Build history of the part. All positions in model axes, mm. A direction names the side the tool comes from. Round coordinates to 2 decimals unless told otherwise and drop trailing zeros. Order: outer loops, then holes, each group sorted by start corner. A loop starts at its lowest first (then second) coordinate and runs counter-clockwise, first axis right, second up. Notation, with made-up numbers: (-21, 84.5) - (3, 84.5) arc R13 ccw to (3, 93.5) - close; hole circle Ø10 at (13, -11.75). An arc over 180 degrees is marked (long way). One line per question, with ' | ' between items. Start each with the question number.
Autodesk Inventor part; units mm, degrees
ref_plane "YZ Plane" through (0, 0, 0) normal (1, 0, 0) x (0, 1, 0)
ref_plane "XZ Plane" through (0, 0, 0) normal (0, 1, 0) x (-1, 0, 0)
ref_plane "XY Plane" through (0, 0, 0) normal (0, 0, 1) x (1, 0, 0)
sketch "Sketch1" plane through (0, 0, 0) normal (0, 1, 0) x (-1, 0, 0)
  circle A0 centre (7.3, 0) radius 1.55
  circle A1 centre (0, 0) radius 1.55
  line L0 (0, 10.8163) -> (0, -10.8163)
  line L1 (6.335, 0) -> (-6.335, 0)
  line L2 (-3.55, 12.16) -> (16.45, 12.16)
  line L3 (16.45, 12.16) -> (16.45, -12.16)
  line L4 (16.45, -12.16) -> (-3.55, -12.16)
  line L5 (-3.55, -12.16) -> (-3.55, 12.16)
  dimension "d0" = 3.1
  dimension "d1" = 7.3
  dimension "d2" = 2
  dimension "d3" = 24.32
  dimension "d4" = 20
extrude "Extrusion1" add sketch "Sketch1" along normal blind 10
sketch "Sketch2" plane through (0, 0, 0) normal (0, -1, 0) x (1, 0, 0)
  line L0 (3.55, 4.76) -> (-11.68, 4.76)
  line L1 (-11.68, 4.76) -> (-11.68, -4.76)
  line L2 (-11.68, -4.76) -> (3.55, -4.76)
  line L3 (3.55, -4.76) -> (3.55, 4.76)
  circle A0 centre (0, 0) radius 1.55
  circle A1 centre (-7.3, 0) radius 1.55
  line L4 (0, 0) -> (-7.3, 0)
  line L5 (3.55, 12.16) -> (3.55, -12.16)
  dimension "d7" = 9.52
  dimension "d8" = 4.38
extrude "Extrusion2" cut sketch "Sketch2" against normal blind 3
sketch "Sketch3" plane through (0, 10, 0) normal (0, 1, 0) x (1, 0, 0)
  circle A0 centre (-7.3, 0) radius 1.55
  circle A1 centre (0, 0) radius 1.55
  arc A2 (3.55, -1.2083) -> (3.55, 1.2083) centre (0, 0) ccw
  arc A3 (-7.3, 3.75) -> (-7.3, -3.75) centre (-7.3, 0) ccw
  line L0 (3.55, -12.16) -> (3.55, 12.16)
  line L1 (-7.3, 3.75) -> (0, 3.75)
  line L2 (-7.3, -3.75) -> (0, -3.75)
  line L3 (3.55, -1.2083) -> (3.55, 1.2083)
  line L4 (3.55, -1.2083) -> (3.55, 1.2083)
  line L5 (0, -3.75) -> (3.55, -3.75)
  line L6 (0, 3.75) -> (3.55, 3.75)
  dimension "d11" = 7.5
extrude "Extrusion3" cut sketch "Sketch3" against normal blind 3 contours L0 L5 L2 A3 L1 L6
sketch "Sketch4" plane through (0, 10, 0) normal (0, 1, 0) x (1, 0, 0)
  line L0 (3.55, -12.16) -> (3.55, -3.75)
  line L1 (3.55, -3.75) -> (-7.3, -3.75)
  arc A0 (-7.3, 3.75) -> (-7.3, -3.75) centre (-7.3, 0) ccw
  line L2 (-7.3, 3.75) -> (3.55, 3.75)
  line L3 (3.55, 3.75) -> (3.55, -3.75)
  circle A1 centre (0, -7.955) radius 1.5
  circle A2 centre (-12.9, -7.955) radius 1.5
  line L4 (-16.45, 12.16) -> (-16.45, -12.16)
  line L5 (-16.45, 0) -> (3.55, 0)
  circle A3 centre (0, 7.955) radius 1.5
  circle A4 centre (-12.9, 7.955) radius 1.5
  line L6 (3.55, -7.955) -> (-16.45, -7.955)
  line L7 (3.55, 4.76) -> (3.55, 12.16)
  line L8 (3.55, 7.955) -> (-16.45, 7.955)
  line L9 (-11.05, 0) -> (-16.45, 0) construction
  point P0 (0, 0)
  dimension "d15" = 3
  dimension "d16" = 3
  dimension "d18" = 3.55
  dimension "d19" = 3.55
extrude "Extrusion4" cut sketch "Sketch4" against normal blind 5 contours L6 A1 | A1 L6 | L6 A2 | A2 L6 | L8 A3 | A3 L8 | L8 A4 | A4 L8
chamfer "Chamfer1" distance 0.5 angle 45 26 edges at (3.55, 10, 7.955) (-1.875, 10, 3.75) (-11.05, 10, 0) (-1.875, 10, -3.75) (3.55, 10, -7.955) (-6.45, 10, -12.16) (-16.45, 10, 0) (-6.45, 10, 12.16) (3.55, 5, 12.16) (3.55, 0, 8.46) (-6.45, 0, 12.16) (-16.45, 0, 0) (-6.45, 0, -12.16) (3.55, 0, -8.46) (3.55, 5, -12.16) (-16.45, 5, -12.16) (-16.45, 5, 12.16) (-11.68, 0, 0) (-4.065, 0, 4.76) (-4.065, 0, -4.76) (3.55, 1.5, 4.76) (3.55, 1.5, -4.76) (3.55, 3, 0) (3.55, 7, 0) (3.55, 8.5, 3.75) (3.55, 8.5, -3.75)
ref_plane "Work Plane1" through (-15.95, 0.5, 0) normal (0, 0, 1) x (1, 0, 0)
equation "\"d0\" = spacer_hole_diameter"
equation "\"d1\" = load_cell_hole_discance"
equation "\"load_cell_hole_discance\" = 7.3"
equation "\"spacer_hole_diameter\" = 3.1"
equation "\"load_cell_width\" = 9.32"
equation "\"load_cell_hole_edge\" = 4.18"
properties part number "load_cell_connector_top"
Item 1: Slice it at B-B (x = -12.9). Write the cut outline in (y, z) (3 decimals).
Item 2: Pin check, flat tips, straight feed: pin 1 (5 mm diameter, centred on x = 0, z = 0, fed in from +Y); pin 2 (2.5 mm diameter, centred on x = 0, z = -7.955, fed in from +Y); pin 3 (4 mm diameter, centred on x = -7.3, z = 0, fed in from -Y). Stop position of each tip, or through.
Item 3: 3-axis set-ups, long thin cutter, end or side, ignore diameter. For faces 4 (the face through (-13, 0, 0)), 5 (the face through (-2, 8, -3.75)), 6 (the face through (-4, 2, -4.76)), 7 (the face through (0, 5, 8)): which of +Z, -Z, +X, -X, +Y, -Y reach the whole face in a straight line?
Item 4: Pull direction Z, two halves, no side cores. Call faces 1 (the face through (-0.715, 4.972, 1.375)), 2 (the face through (-6, 5, 12.16)), 3 (the face through (3.55, 5, 0)): released by +Z, released by -Z, zero draft, split by the parting line, or undercut.
Item 5: Slice it at A-A (z = 0). Write the cut outline in (x, y).
Item 6: Wall check: line 1 along Z through (x, y) = (-12.9, 6.65) (3 decimals); line 2 along X through (y, z) = (4.2, 0); line 3 along Z through (x, y) = (0, 7.85) (3 decimals). Give the ranges that are in metal, low to high. Write a range as [from, to].
Item 7: Slice it at D-D (z = 6.75). Write the cut outline in (x, y), plus the area to 3 significant figures.
A:
1) outline: (0, -11.66) - (0.5, -12.16) - (9.5, -12.16) - (10, -11.66) - (10, -9.455) - (5, -9.455) - (5, -6.455) - (10, -6.455) - (10, 6.455) - (5, 6.455) - (5, 9.455) - (10, 9.455) - (10, 11.66) - (9.5, 12.16) - (0.5, 12.16) - (0, 11.66) - close
2) pin 1: y = 7 | pin 2: y = 5 | pin 3: y = 3
3) face 4: +Z, -Z, +X, -X, -Y | face 5: +X, +Y | face 6: +X, -Y | face 7: +Y
4) face 1: undercut | face 2: released by +Z | face 3: zero draft
5) outline: (-16.45, 0.5) - (-15.95, 0) - (-12.18, 0) - (-11.68, 0.5) - (-11.68, 3) - (-8.85, 3) - (-8.85, 7) - (-11.05, 7) - (-11.05, 9.5) - (-11.55, 10) - (-15.95, 10) - (-16.45, 9.5) - close; (-5.75, 3) - (-1.55, 3) - (-1.55, 7) - (-5.75, 7) - close; (1.55, 3) - (3.05, 3) - (3.55, 3.5) - (3.55, 6.5) - (3.05, 7) - (1.55, 7) - close
6) line 1: [-12.16, -9.455], [-6.455, 6.455], [9.455, 12.16] | line 2: [-16.45, -8.85], [-5.75, -1.55], [1.55, 3.55] | line 3: [-12.16, -9.455], [-6.455, -3.75], [3.75, 6.455], [9.455, 12.16]
7) outline: (-16.45, 0.5) - (-15.95, 0) - (3.05, 0) - (3.55, 0.5) - (3.55, 9.5) - (3.05, 10) - (0.89, 10) - (0.89, 5) - (-0.89, 5) - (-0.89, 10) - (-12.01, 10) - (-12.01, 5) - (-13.79, 5) - (-13.79, 10) - (-15.95, 10) - (-16.45, 9.5) - close | area: 182 mm^2
